Source: CAD feature listing. Evaluate the final solid. Frame: model axes, mm. Give positions to 0.01 mm unless a question says otherwise; leave off trailing zeros. Loops run counter-clockwise (first coordinate to the right, second up) from the corner with the lowest first, then second, coordinate; pieces in that order, holes last. Notation, with made-up numbers: (80.5, -11.75) -> (128.5, -11.75) arc R15 cw to (128.5, 7.25) -> close; hole circle Ø9 at (18, 72.25). An arc over 180 degrees is marked (long way). Return JSON: item names as keys, results as strings. Group by question number.
(1) Cut plane A-A on z = 76.2. Return loops of the section in (x, y), then the cut area to 3 significant figures.
(2) Ray query, line 1 (Z direction, x = -1.5, y = -16.5); line 2 (Z direction, x = -25.4, y = -6); line 3 (X direction, y = -21.75, z = 4.5). Return the intervals inside material, ascending. Write a range as from..to.
(3) Pin query (flat end, axial travel): pin 1 (1.5 mm diameter, centred on x = 93.5, y = -16.5, fed in from -Z); pin 2 (4 mm diameter, centred on x = -15.5, y = -15, fed in from -Z); pin 3 (10 mm diameter, centred on y = -11.5, z = -20.5, fed in from -X); pin 4 (5.5 mm diameter, centred on x = -39.14, z = 7.03, fed in from -Y). Return the tip coordinate at first contact, or that it passes through.
(4) Cut plane C-C on x = -132.5. Return loops of the section in (y, z).
(5) Cut plane B-B on y = -6.75. Return loops of the section in (x, z).
(6) Cut plane D-D on z = -97. Return loops of the section in (x, y), then the cut area to 3 significant figures.
(7) Draft query along Z for faces 1 (the face through (-29.82, -13.98, 67.7)), 2 (the face through (-23.449, -6.606, 67.414)), 3 (the face through (-2, 0, 2)), 4 (the face through (-37.116, -12.522, -167.145)). Return one class per face: released by +Z, released by -Z, zero draft, split by the parting line, or undercut.
```python
from build123d import *

# Parameters (mm, degrees)
F0_R           = 171.216465226
F1_DEPTH       = 25.4
F3_D           = 8.8
F4_D           = 18
F4_CSINK_D     = 42
F4_CSINK_ANGLE = 90
F5_D           = 4.1
F5_DEPTH       = 12.7
F5_CSINK_D     = 15.2
F5_CSINK_ANGLE = 90
F5_TIP         = 1.231764269


with BuildPart() as f1:
    # F0 (on Front) → F1 (new body)
    with BuildSketch(Plane.XZ):
        Circle(F0_R)
    extrude(amount=F1_DEPTH)

    # F3 (through all)
    with Locations(Plane.XZ.offset(25.4)):
        with Locations((-39.1375060386, 7.0279744302)):
            Hole(F3_D / 2)

    # F4 (through all)
    with Locations(Plane.XZ.offset(25.4)):
        with Locations((-25.4, 76.2)):
            CounterSinkHole(F4_D / 2, F4_CSINK_D / 2, counter_sink_angle=F4_CSINK_ANGLE)

    # F5
    with Locations(Plane.XZ.offset(25.4)):
        with Locations((-16.2783094505, -23.9721943216)):
            CounterSinkHole(F5_D / 2, F5_CSINK_D / 2, depth=F5_DEPTH, counter_sink_angle=F5_CSINK_ANGLE)
            with Locations((0, 0, -(F5_DEPTH + F5_TIP / 2))):  # 118° drill point
                Cone(0, F5_D / 2, F5_TIP, mode=Mode.SUBTRACT)


solid = f1.part
```
Answers:
{
 "1": {"outline": "(-153.33, -25.4) -> (-46.4, -25.4) -> (-34.4, -13.4) -> (-34.4, 0) -> (-153.33, 0) -> close; (-16.4, -13.4) -> (-4.4, -25.4) -> (153.33, -25.4) -> (153.33, 0) -> (-16.4, 0) -> close", "area": "7,190 mm²"},
 "2": {"line 1": "-171.21..171.21", "line 2": "-169.32..67.2, 85.2..169.32", "line 3": "-171.16..-42.74, -35.54..171.16"},
 "3": {"pin 1": "z = -143.92", "pin 2": "z = -170.68", "pin 3": "x = -170.51", "pin 4": "through"},
 "4": {"outline": "(-25.4, -108.44) -> (0, -108.44) -> (0, 108.44) -> (-25.4, 108.44) -> close"},
 "5": {"outline": "circle Ø342.43 at (0, 0); hole circle Ø8.8 at (-39.14, 7.03); hole circle Ø18 at (-25.4, 76.2)"},
 "6": {"outline": "(-141.09, -25.4) -> (141.09, -25.4) -> (141.09, 0) -> (-141.09, 0) -> close", "area": "7,170 mm²"},
 "7": {"face 1": "undercut", "face 2": "undercut", "face 3": "zero draft", "face 4": "split by the parting line"}
}
